from build123d import *

# Parameters (mm, degrees)
F0_R     = 10.9982
F0_R_2   = 10.9137143354
F1_DEPTH = 12.7


with BuildPart() as f1:
    # F0 (on Top) → F1 (new body)
    with BuildSketch(Plane.XY):
        with BuildLine():
            ThreePointArc((-25.8441113636, 12.9163114686), (-36.6183263022, 12.8623681815), (-44.1497681666, 5.1575644288))
            ThreePointArc((-44.1497681666, 5.1575644288), (-44.45, 0), (-44.1497681666, -5.1575644288))
            ThreePointArc((-44.1497681666, -5.1575644288), (-34.8282447282, -13.4816128788), (-22.5765010853, -11.016788439))
            ThreePointArc((-22.5765010853, -11.016788439), (-18.6134833709, -6.13009055), (-17.1966857451, 0))
            ThreePointArc((-17.1966857451, 0), (-19.5581271759, 7.7718895994), (-25.8441113636, 12.9163114686))
        make_face()
        with Locations((-31.1666857451, 0)):
            Circle(F0_R, mode=Mode.SUBTRACT)
        with BuildLine():
            ThreePointArc((13.7226451188, -2.6172334521), (13.4752902377, 0), (13.7226451188, 2.6172334521))
            ThreePointArc((13.7226451188, 2.6172334521), (-13.97, 0), (13.7226451188, -2.6172334521))
        make_face()
        Circle(F0_R_2, mode=Mode.SUBTRACT)
        with BuildLine():
            ThreePointArc((41.4152902377, 0), (34.9539662549, 11.7805214005), (21.5469030554, 12.6637249121))
            ThreePointArc((21.5469030554, 12.6637249121), (16.4235288175, 8.583803073), (13.7226451188, 2.6172334521))
            ThreePointArc((13.7226451188, 2.6172334521), (13.9080238048, 1.3144481142), (13.97, 0))
            ThreePointArc((13.97, 0), (13.9080238048, -1.3144481142), (13.7226451188, -2.6172334521))
            ThreePointArc((13.7226451188, -2.6172334521), (16.4235288175, -8.583803073), (21.5469030554, -12.6637249121))
            ThreePointArc((21.5469030554, -12.6637249121), (34.9539662549, -11.7805214005), (41.4152902377, 0))
        make_face()
        with Locations((27.4452902377, 0)):
            Circle(F0_R, mode=Mode.SUBTRACT)
        with BuildLine():
            ThreePointArc((21.5469030554, 12.6637249121), (-2.1118543996, 19.6851125626), (-25.8441113636, 12.9163114686))
            ThreePointArc((-25.8441113636, 12.9163114686), (-19.5581271759, 7.7718895994), (-17.1966857451, 0))
            ThreePointArc((-17.1966857451, 0), (-18.6134833709, -6.13009055), (-22.5765010853, -11.016788439))
            ThreePointArc((-22.5765010853, -11.016788439), (-0.9182159345, -22.6482799794), (21.5469030554, -12.6637249121))
            ThreePointArc((21.5469030554, -12.6637249121), (16.4235288175, -8.583803073), (13.7226451188, -2.6172334521))
            ThreePointArc((13.7226451188, -2.6172334521), (-13.97, 0), (13.7226451188, 2.6172334521))
            ThreePointArc((13.7226451188, 2.6172334521), (16.4235288175, 8.583803073), (21.5469030554, 12.6637249121))
        make_face()
    extrude(amount=F1_DEPTH)


solid = f1.part
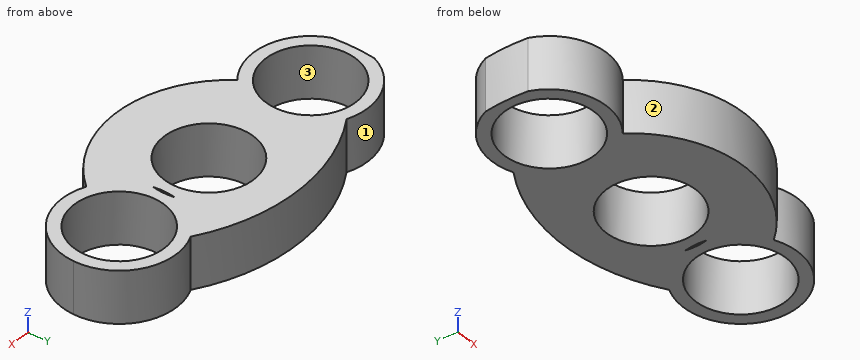
Input: part model. Units: mm. Frame: model coordinates. Face numbers are marked on the shaded views. Coordinates: 2 decimals unless noted, no trailing zeros. Order: outer loops, then holes, each group sorted by start corner. A loop starts at its lowest first (then second) coordinate and runs counter-clockwise, first axis right, second up. Notation, with made-up numbers: M 54.5,-36 L 108.5,-36 A19 ccw 108.5,-21 Z; hole C 64.5,37 d3. An arc over 180 degrees is marked long. Answer in a Markdown table with one row per item.
(1) Section query D-D, the plane x = -39. Output: boundary loops of the cut face in (y, z).
Numbers:
| item | result |
|---|---|
| outline | M -11.57,0 L -7.72,0 L -7.72,12.7 L -11.57,12.7 Z; M 7.72,0 L 11.57,0 L 11.57,12.7 L 7.72,12.7 Z |
(2) Section query A-A, the plane x = 34.5. Output: boundary loops of the cut face in (y, z).
Numbers:
| item | result |
|---|---|
| outline | M -12.06,0 L -8.44,0 L -8.44,12.7 L -12.06,12.7 Z; M 8.44,0 L 12.06,0 L 12.06,12.7 L 8.44,12.7 Z |
(3) Section query C-C, the plane y = -1.5. Output: boundary loops of the cut face in (x, z), plus the area to 3 significant figures.
Numbers:
| item | result |
|---|---|
| outline | M -44.42,0 L -42.06,0 L -42.06,12.7 L -44.42,12.7 Z; M -20.27,0 L -10.81,0 L -10.81,12.7 L -20.27,12.7 Z; M 10.81,0 L 13.56,0 L 13.56,12.7 L 10.81,12.7 Z; M 13.89,0 L 16.55,0 L 16.55,12.7 L 13.89,12.7 Z; M 38.34,0 L 41.33,0 L 41.33,12.7 L 38.34,12.7 Z |
| area | 257 mm^2 |
(4) Section query B-B, the plane z = 2.25. Output: boundary loops of the cut face in (x, y).
Numbers:
| item | result |
|---|---|
| outline | M -44.15,-5.16 A13.97 ccw -22.58,-11.02 A27.94 ccw 21.55,-12.66 A13.97 ccw long 21.55,12.66 A44.16 ccw -25.84,12.92 A13.97 ccw -44.15,5.16 A44.45 ccw Z; hole C -31.17,0 d22; hole C 0,0 d21.83; hole M 13.72,-2.62 A13.97 ccw 13.72,2.62 A13.97 ccw Z; hole C 27.45,0 d22 |
(5) Material intervals for line 1 (X direction, y = 0.5, z = 3); line 2 (X direction, y = 6, z = 1.25); line 3 (Y direction, x = -1.5, z = 6.5), sorted ascending. Write a range as [from, to].
Numbers:
| item | result |
|---|---|
| line 1 | x = [-44.45, -42.15], [-20.18, -10.9], [10.9, 13.48], [13.96, 16.46], [38.43, 41.41] |
| line 2 | x = [-43.78, -40.38], [-21.95, -9.12], [9.12, 18.23], [36.66, 40.06] |
| line 3 | y = [-22.62, -10.81], [10.81, 19.68] |
(6) Draft query along Y for the marked faces 1, 2 and 3. Return one class per face: pulls with the +Y half, pulls with the -Y half, needs draft (parallel to the pull), parting line crosses it, or undercut.
Numbers:
| item | result |
|---|---|
| face 1 | pulls with the +Y half |
| face 2 | pulls with the -Y half |
| face 3 | undercut |
(7) Contact query for flat-ended pins moving along their axis: pin 1 Ø25 at (x, y) = (0, 0) entering from -Z; pin 2 Ø4 at (y, z) = (6, 3.5) entering from +X; pin 3 Ø6 at (y, z) = (9, 9) entering from +X; pin 4 Ø1.5 at (x, z) = (-28, 6) entering from +Y. Output: stop coordinate, or through.
Numbers:
| item | result |
|---|---|
| pin 1 | stops at z = 0 |
| pin 2 | stops at x = 40.83 |
| pin 3 | stops at x = 40.06 |
| pin 4 | stops at y = 13.76 |
